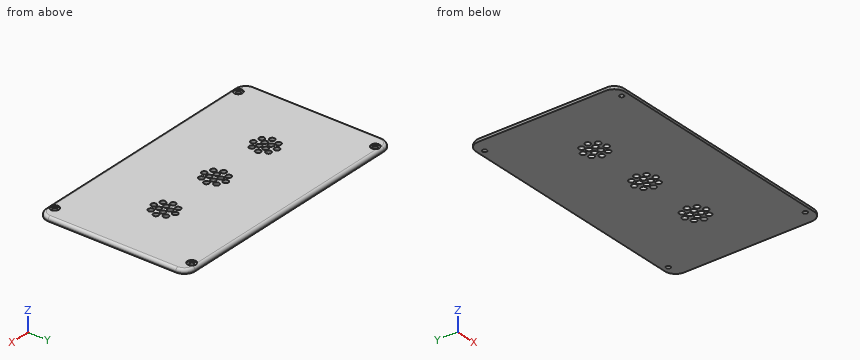
Autodesk Fusion 360 part; units mm, degrees
sketch "Sketch1" plane through (0, 0, 0) normal (0, 0, 1) x (1, 0, 0)
  line L0 (8, 0) -> (185, 0)
  line L1 (193, 8) -> (193, 103)
  line L2 (185, 111) -> (8, 111)
  line L3 (0, 103) -> (0, 8)
  arc A0 (8, 111) -> (0, 103) centre (8, 103) ccw
  arc A1 (193, 103) -> (185, 111) centre (185, 103) ccw
  arc A2 (185, 0) -> (193, 8) centre (185, 8) ccw
  arc A3 (0, 8) -> (8, 0) centre (8, 8) ccw
  point P0 (193, 0)
  point P1 (0, 111)
  dimension "d1" = 193
  dimension "d2" = 111
  dimension "d3" = 8
  dimension "d4" = 8
  dimension "d5" = 8
  dimension "d6" = 8
extrude "Extrude1" add sketch "Sketch1" along normal blind 3
fillet "Fillet1" radius 2 8 edges at (193, 55.5, 3) (190.6569, 108.6569, 3) (96.5, 111, 3) (2.3431, 108.6569, 3) (0, 55.5, 3) (2.3431, 2.3431, 3) (96.5, 0, 3) (190.6569, 2.3431, 3)
sketch "Sketch2" plane through (0, 0, 3) normal (0, 0, 1) x (-1, 0, 0)
  line L0 (-191, -8) -> (-191, -103)
  arc A0 (-191, -103) -> (-185, -109) centre (-185, -103) ccw
  line L1 (-185, -109) -> (-8, -109)
  arc A1 (-8, -109) -> (-2, -103) centre (-8, -103) ccw
  line L2 (-2, -103) -> (-2, -8)
  arc A2 (-2, -8) -> (-8, -2) centre (-8, -8) ccw
  line L3 (-8, -2) -> (-185, -2)
  arc A3 (-185, -2) -> (-191, -8) centre (-185, -8) ccw
  line L4 (-8, -109) -> (-13, -109)
  line L5 (-13, -109) -> (-13, -104)
  line L6 (-13, -104) -> (-8, -104)
  line L7 (-8, -104) -> (-8, -109)
  circle A4 centre (-10.5, -106.5) radius 1.6
  line L8 (-185, -109) -> (-180, -109)
  line L9 (-180, -109) -> (-180, -104)
  line L10 (-180, -104) -> (-185, -104)
  line L11 (-185, -104) -> (-185, -109)
  circle A5 centre (-182.5, -106.5) radius 1.6
  line L12 (-185, -2) -> (-180, -2)
  line L13 (-180, -2) -> (-180, -7)
  line L14 (-180, -7) -> (-185, -7)
  line L15 (-185, -7) -> (-185, -2)
  circle A6 centre (-182.5, -4.5) radius 1.6
  line L16 (-8, -2) -> (-13, -2)
  line L17 (-13, -2) -> (-13, -7)
  line L18 (-13, -7) -> (-8, -7)
  line L19 (-8, -7) -> (-8, -2)
  circle A7 centre (-10.5, -4.5) radius 1.6
  point P0 (-10.5, -106.5)
  dimension "d11" = 5
  dimension "d12" = 5
  dimension "d13" = 3.2
  dimension "d14" = 5
  dimension "d15" = 5
  dimension "d16" = 3.2
  dimension "d17" = 5
  dimension "d18" = 5
  dimension "d19" = 3.2
  dimension "d20" = 5
  dimension "d21" = 5
  dimension "d22" = 3.2
hole "Hole1" at (10.5, 4.5, 3) at (10.5, 106.5, 3) at (182.5, 106.5, 3) at (182.5, 4.5, 3) direction (0, 0, -1) diameter 3.2 depth 7 tip angle 180
sketch "Sketch3" plane through (0, 0, 3) normal (0, 0, 1) x (-1, 0, 0)
  circle A0 centre (-182.5, -106.5) radius 1.6
  circle A1 centre (-10.5, -4.5) radius 1.6
  circle A2 centre (-10.5, -106.5) radius 1.6
  circle A3 centre (-182.5, -4.5) radius 1.6
  line L0 (-191, -8) -> (-191, -103)
  arc A4 (-191, -103) -> (-185, -109) centre (-185, -103) ccw
  line L1 (-185, -109) -> (-8, -109)
  arc A5 (-8, -109) -> (-2, -103) centre (-8, -103) ccw
  line L2 (-2, -103) -> (-2, -8)
  arc A6 (-2, -8) -> (-8, -2) centre (-8, -8) ccw
  line L3 (-8, -2) -> (-185, -2)
  arc A7 (-185, -2) -> (-191, -8) centre (-185, -8) ccw
  circle A8 centre (-10.5, -106.5) radius 3.2
  circle A9 centre (-182.5, -106.5) radius 3.2
  circle A10 centre (-182.5, -4.5) radius 3.2
  circle A11 centre (-10.5, -4.5) radius 3.2
  dimension "d26" = 6.4
  dimension "d27" = 6.4
  dimension "d28" = 6.4
  dimension "d29" = 6.4
hole "Hole2" at (182.5, 4.5, 3) at (10.5, 4.5, 3) at (182.5, 106.5, 3) at (10.5, 106.5, 3) direction (0, 0, -1) diameter 6.4 depth 0.854 tip angle 180
sketch "Sketch4" plane through (0, 0, 3) normal (0, 0, 1) x (-1, 0, 0)
  arc A0 (-180.5025, -109) -> (-184.4975, -109) centre (-182.5, -106.5) ccw
  line L0 (-180.5025, -109) -> (-12.4975, -109)
  arc A1 (-8.5025, -109) -> (-12.4975, -109) centre (-10.5, -106.5) ccw
  line L1 (-8.5025, -109) -> (-8, -109)
  arc A2 (-8, -109) -> (-2, -103) centre (-8, -103) ccw
  line L2 (-2, -103) -> (-2, -8)
  arc A3 (-2, -8) -> (-8, -2) centre (-8, -8) ccw
  line L3 (-8, -2) -> (-8.5025, -2)
  arc A4 (-12.4975, -2) -> (-8.5025, -2) centre (-10.5, -4.5) ccw
  line L4 (-12.4975, -2) -> (-180.5025, -2)
  arc A5 (-184.4975, -2) -> (-180.5025, -2) centre (-182.5, -4.5) ccw
  line L5 (-184.4975, -2) -> (-185, -2)
  arc A6 (-185, -2) -> (-191, -8) centre (-185, -8) ccw
  line L6 (-191, -8) -> (-191, -103)
  arc A7 (-191, -103) -> (-185, -109) centre (-185, -103) ccw
  line L7 (-185, -109) -> (-184.4975, -109)
  circle A8 centre (-41.5919, -54.4399) radius 2
  circle A9 centre (-44.664, -49.1434) radius 2
  circle A10 centre (-50.5814, -47.5705) radius 2
  circle A11 centre (-55.8779, -50.6426) radius 2
  circle A12 centre (-57.4508, -56.5601) radius 2
  circle A13 centre (-54.3787, -61.8566) radius 2
  circle A14 centre (-48.4612, -63.4295) radius 2
  circle A15 centre (-43.1648, -60.3574) radius 2
  circle A16 centre (-46.9732, -53.1006) radius 2
  circle A17 centre (-51.9207, -52.9519) radius 2
  circle A18 centre (-52.0695, -57.8994) radius 2
  circle A19 centre (-47.122, -58.0481) radius 2
  circle A20 centre (-95.1603, -58.7335) radius 2
  circle A21 centre (-96.5061, -47.5) radius 2
  circle A22 centre (-102.1612, -49.8474) radius 2
  circle A23 centre (-96.4939, -63.5) radius 2
  circle A24 centre (-104.5, -55.5061) radius 2
  circle A25 centre (-93.2665, -54.1603) radius 2
  circle A26 centre (-99.7335, -56.8397) radius 2
  circle A27 centre (-90.8474, -49.8388) radius 2
  circle A28 centre (-90.8388, -61.1526) radius 2
  circle A29 centre (-97.8397, -52.2665) radius 2
  circle A30 centre (-102.1526, -61.1612) radius 2
  circle A31 centre (-88.5, -55.4939) radius 2
  circle A32 centre (-147.0416, -56.8385) radius 2
  circle A33 centre (-151.8076, -55.479) radius 2
  circle A34 centre (-142.4691, -58.734) radius 2
  circle A35 centre (-138.1359, -49.858) radius 2
  circle A36 centre (-138.1656, -61.1717) radius 2
  circle A37 centre (-143.8286, -63.5) radius 2
  circle A38 centre (-143.7866, -47.5) radius 2
  circle A39 centre (-149.4793, -61.142) radius 2
  circle A40 centre (-149.4496, -49.8283) radius 2
  circle A41 centre (-145.1461, -52.266) radius 2
  circle A42 centre (-135.8076, -55.521) radius 2
  circle A43 centre (-140.5736, -54.1615) radius 2
  point P0 (-49.5213, -55.5)
  point P1 (-96.5, -55.5)
  point P2 (-143.8076, -55.5)
  dimension "d33" = 8
  dimension "d34" = 4
  dimension "d37" = 360
  dimension "d40" = 3.5
  dimension "d41" = 4
  dimension "d43" = 360
  dimension "d45" = 360
  dimension "d47" = 360
  dimension "d48" = 8
  dimension "d49" = 4
  dimension "d50" = 3.5
  dimension "d51" = 4
  dimension "d55" = 360
  dimension "d57" = 360
  dimension "d58" = 8
  dimension "d59" = 4
  dimension "d60" = 3.5
  dimension "d61" = 4
hole "Hole3" at (52.0695, 57.8994, 3) at (47.122, 58.0481, 3) at (48.4612, 63.4295, 3) at (43.1648, 60.3574, 3) at (41.5919, 54.4399, 3) at (46.9732, 53.1006, 3) at (44.664, 49.1434, 3) at (55.8779, 50.6426, 3) at (51.9207, 52.9519, 3) at (50.5814, 47.5705, 3) at (57.4508, 56.5601, 3) at (54.3787, 61.8566, 3) at (96.4939, 63.5, 3) at (90.8388, 61.1526, 3) at (88.5, 55.4939, 3) at (95.1603, 58.7335, 3) at (93.2665, 54.1603, 3) at (97.8397, 52.2665, 3) at (90.8474, 49.8388, 3) at (96.5061, 47.5, 3) at (102.1612, 49.8474, 3) at (102.1526, 61.1612, 3) at (104.5, 55.5061, 3) at (99.7335, 56.8397, 3) at (142.4691, 58.734, 3) at (138.1656, 61.1717, 3) at (143.8286, 63.5, 3) at (149.4793, 61.142, 3) at (147.0416, 56.8385, 3) at (149.4496, 49.8283, 3) at (145.1461, 52.266, 3) at (151.8076, 55.479, 3) at (143.7866, 47.5, 3) at (138.1359, 49.858, 3) at (140.5736, 54.1615, 3) at (135.8076, 55.521, 3) direction (0, 0, -1) diameter 4 depth 10 tip angle 180
Verification items for the finished model (mm, model axes). Coordinates: 2 decimals unless noted, no trailing zeros. Write item = value, one per line.
Q1. Material ranges on L1, parallel to Y at x = 10.5, z = 1.6; L2, parallel to Y at x = 9.5, z = 1.55; L3, parallel to Y at x = 96, z = 0.25, recorded low to high. Write a range as from..to.
Answer:
L1 = 0.09..2.9, 6.1..104.9, 108.1..110.91
L2 = 0.08..3.25, 5.75..105.25, 107.75..110.92
L3 = 0..45.57, 49.43..51.48, 53.05..56.92, 60.55..61.56, 65.44..111
Q2. Go/stop test with flat-tipped pins: pin 1 Ø1.9 at (x, y) = (181.5, 108) entering from +Z; pin 2 Ø2.5 at (x, y) = (143.79, 47.5) entering from -Z; pin 3 Ø1.5 at (y, z) = (47.5, 2.5) entering from -X. Record where each tip stops, or that it passes through.
Answer:
pin_1 = 2.15
pin_2 = through
pin_3 = 0.15
Q3. Cross-section at A-A (z = 1.5). Give the number of separate pieces and of enclosed holes in the cut face, plus the area to 3 significant figures.
Answer:
separate_pieces = 1
enclosed_holes = 40
area = 20,800 mm²
